Source: CAD feature listing. Evaluate the final solid. Frame: model axes, mm. A direction names the side the tool comes from. Coordinates: 2 decimals unless noted, no trailing zeros. Order: outer loops, then holes, each group sorted by start corner. A loop starts at its lowest first (then second) coordinate and runs counter-clockwise, first axis right, second up. Notation, with made-up numbers: (-20.5, 19) -> (-15.5, 19) arc R15 cw to (-15.5, 27) -> close; hole circle Ø3 at (-23.75, -30.5). An arc over 180 degrees is marked (long way). Write item = value, one per line. Start each with the question number.
Item 1: Section query D-D (z = -1.5). Output: boundary loops of the cut face in (x, y).
Item 2: Set-up query: faces 4 (the flat face through (0, 0, -8)), 5 (the flat face through (0, -5, 0)), 6 (the flat face through (-2.04, 1, -6)). Return all of +Z, -Z, +X, -X, +Y, -Y with unobstructed straight access to the full face (end or side cutting, diameter ignored); none if empty.
Item 3: Section query A-A (z = -6). Output: boundary loops of the cut face in (x, y).
Item 4: Ray query, line 1 along Y through (x, z) = (-2.25, -5.25); line 2 along Z through (x, y) = (-3.5, -5); line 3 along Y through (x, z) = (1, -6.75). Return the intervals inside material, ascending. Write a range as [from, to].
Item 5: Section query B-B (x = -1.5). Output: boundary loops of the cut face in (y, z), then the cut area to 3 significant figures.
Item 6: Section query C-C (y = -4.5). Output: boundary loops of the cut face in (x, z).
Item 7: Mould query, pull axis X, two halves, no side actions, for faces 1 (the flat face through (0, 5, 0)), 2 (the flat face through (-2.5, -0.77, -5.5)), 3 (the flat face through (-4, 0, -2)). Classes: released by +X, released by -X, zero draft, split by the parting line, or undercut.
Item 8: Contact query for flat-ended pins moving along their axis: pin 1 (0.8 mm diameter, centred on x = 0, z = -5.5, fed in from +Y); pin 2 (2 mm diameter, centred on x = 2.5, z = -6.5, fed in from -Y); pin 3 (1.5 mm diameter, centred on x = 0, y = -4.5, fed in from -Z); pin 4 (1.1 mm diameter, centred on x = 2.5, y = -1.5, fed in from -Z). Output: stop coordinate, or through.
```python
from build123d import *

# Parameters (mm, degrees)
SKETCH002_W  = 15
SKETCH002_H  = 1.6
PAD001_DEPTH = 4
SKETCH_W     = 5
SKETCH_H     = 8
PAD_DEPTH    = 4
SKETCH001_W  = 1
SKETCH001_H  = 1
POCKET_DEPTH = 5


with BuildPart() as pad001:
    # Sketch002 → Pad001 (new body, symmetric)
    with BuildSketch(Plane.YZ):
        with Locations((0, 0.8)):
            Rectangle(SKETCH002_W, SKETCH002_H)
    extrude(amount=PAD001_DEPTH, both=True)


with BuildPart() as fusion:
    # Sketch → Pad (new body, symmetric)
    with BuildSketch(Plane.YZ):
        with Locations((0, -4)):
            Rectangle(SKETCH_W, SKETCH_H)
    extrude(amount=PAD_DEPTH, both=True)

    # Sketch001 → Pocket (cut)
    with BuildSketch(Plane.YX.offset(8)):
        with Locations((-1.27, 2.54)):
            Rectangle(SKETCH001_W, SKETCH001_H)
        with Locations((1.27, 2.54)):
            Rectangle(SKETCH001_W, SKETCH001_H)
        with Locations((-1.27, 0)):
            Rectangle(SKETCH001_W, SKETCH001_H)
        with Locations((1.27, 0)):
            Rectangle(SKETCH001_W, SKETCH001_H)
        with Locations((-1.27, -2.54)):
            Rectangle(SKETCH001_W, SKETCH001_H)
        with Locations((1.27, -2.54)):
            Rectangle(SKETCH001_W, SKETCH001_H)
    extrude(amount=-POCKET_DEPTH, mode=Mode.SUBTRACT)

    # Fusion: union Pad001
    add(pad001.part)


solid = fusion.part
```
Computed:
q1.outline = (-4, -2.5) -> (4, -2.5) -> (4, 2.5) -> (-4, 2.5) -> close
q2.face_4 = -Z, +X, -X, +Y, -Y
q2.face_5 = -Z, +X, -X, -Y
q2.face_6 = -Z
q3.outline = (-4, -2.5) -> (4, -2.5) -> (4, 2.5) -> (-4, 2.5) -> close; hole (-3.04, -1.77) -> (-2.04, -1.77) -> (-2.04, -0.77) -> (-3.04, -0.77) -> close; hole (-3.04, 0.77) -> (-2.04, 0.77) -> (-2.04, 1.77) -> (-3.04, 1.77) -> close; hole (-0.5, -1.77) -> (0.5, -1.77) -> (0.5, -0.77) -> (-0.5, -0.77) -> close; hole (-0.5, 0.77) -> (0.5, 0.77) -> (0.5, 1.77) -> (-0.5, 1.77) -> close; hole (2.04, -1.77) -> (3.04, -1.77) -> (3.04, -0.77) -> (2.04, -0.77) -> close; hole (2.04, 0.77) -> (3.04, 0.77) -> (3.04, 1.77) -> (2.04, 1.77) -> close
q4.line_1 = [-2.5, -1.77], [-0.77, 0.77], [1.77, 2.5]
q4.line_2 = [0, 1.6]
q4.line_3 = [-2.5, 2.5]
q5.outline = (-7.5, 0) -> (-2.5, 0) -> (-2.5, -8) -> (2.5, -8) -> (2.5, 0) -> (7.5, 0) -> (7.5, 1.6) -> (-7.5, 1.6) -> close
q5.area = 64.0 mm^2
q6.outline = (-4, 0) -> (4, 0) -> (4, 1.6) -> (-4, 1.6) -> close
q7.face_1 = zero draft
q7.face_2 = undercut
q7.face_3 = released by -X
q8.pin_1 = 2.5
q8.pin_2 = -2.5
q8.pin_3 = 0
q8.pin_4 = -8
